Could you check a few things on this drawing? It's one solid part, dimensions in mm from its lowest x, y, z. Give positions to 0.01 mm unless a question says otherwise; leave off trailing zeros. Write each loop counter-clockwise with the first axis right and the second up, starting at its lowest first coordinate (ties: lowest second). Pieces come first, ordered by that corner, then holes. Notation, with made-up numbers: M -28.5,51 L 4.5,51 A36 ccw 4.5,87 Z; hole C -6.75,54 d2. An arc over 180 degrees is marked long. Use CSV: the item, a comma, the result in double quotes. Start each with the question number.
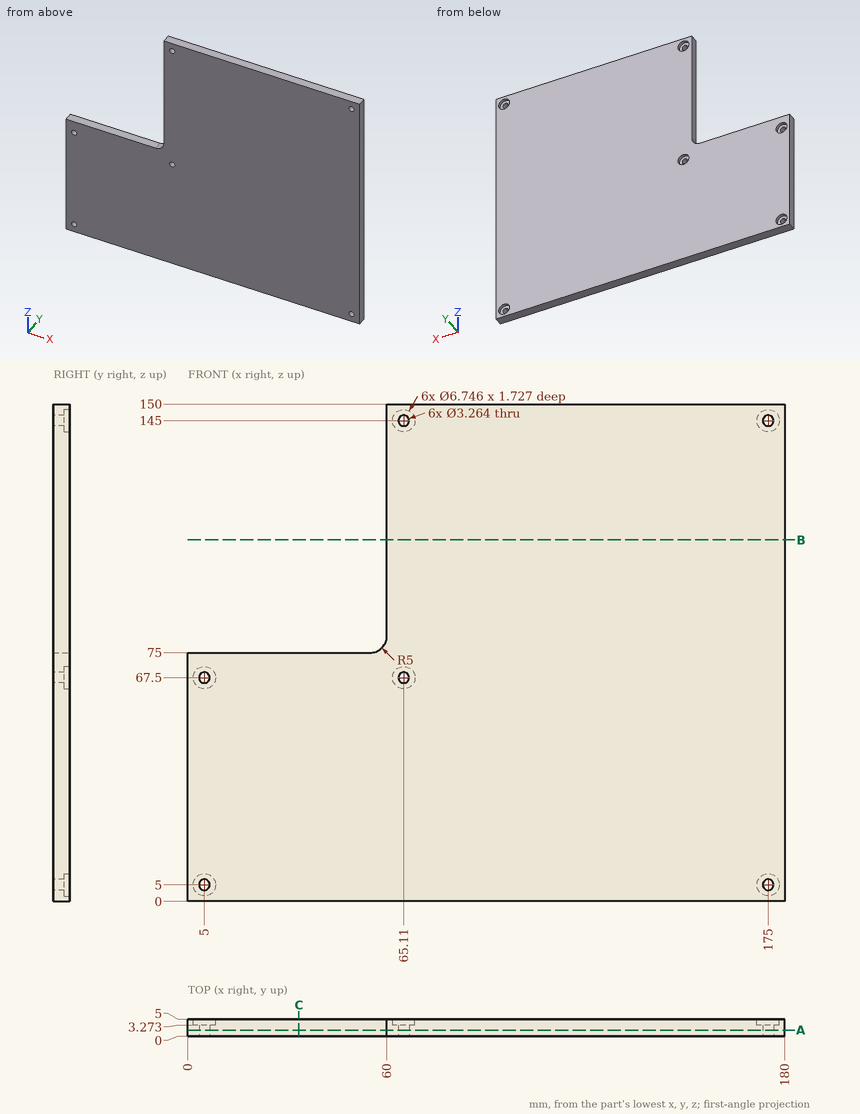
(1) I want a section at B-B (z = 109). Write out the boundary of the cut face in (x, y), and give its area (3 significant figures).
(2) I want a section at A-A (y = 1.75). Write out the boundary of the cut face in (x, z).
(3) Will these pins go through, and if not, where does the flat tip stop? pin 1 Ø4 at (x, z) = (5, 5) entering from +Y; pin 2 Ø2 at (y, z) = (1.5, 80.5) entering from -X (3 decimals).
(4) I want a section at C-C (x = 33.5). Write out the boundary of the cut face in (y, z), and give its area (3 significant figures).
(5) Please list where these lines run through material, in increasing order: L1, parallel to X at y = 2.45, z = 67.5; L2, parallel to Z at x = 175, y = 2.05; L3, parallel to X at y = 1.45, z = 145. Write a range as [from, to].
Geometry results:
1,outline,"M 60,0 L 180,0 L 180,5 L 60,5 Z"
1,area,"600 mm2"
2,outline,"M 0,0 L 180,0 L 180,150 L 60,150 L 60,80 A5 cw 55,75 L 0,75 Z; hole C 5,5 d3.26; hole C 5,67.5 d3.26; hole C 65.11,67.5 d3.26; hole C 65.11,145 d3.26; hole C 175,5 d3.26; hole C 175,145 d3.26"
3,pin 1,"stops at y = 3.27"
3,pin 2,"stops at x = 59.975"
4,outline,"M 0,0 L 5,0 L 5,75 L 0,75 Z"
4,area,"375 mm2"
5,L1,"x = [0, 3.37], [6.63, 63.48], [66.74, 180]"
5,L2,"z = [0, 3.37], [6.63, 143.37], [146.63, 150]"
5,L3,"x = [60, 63.48], [66.74, 173.37], [176.63, 180]"
